Autodesk Inventor part; units mm, degrees
ref_plane "YZ Plane" through (0, 0, 0) normal (1, 0, 0) x (0, 1, 0)
ref_plane "XZ Plane" through (0, 0, 0) normal (0, 1, 0) x (-1, 0, 0)
ref_plane "XY Plane" through (0, 0, 0) normal (0, 0, 1) x (1, 0, 0)
sketch "Sketch1" plane through (0, 0, 0) normal (0, 0, 1) x (1, 0, 0)
  line L0 (1, -38.4) -> (1, -34.6)
  line L1 (1, -38.4) -> (20.6442, -38.4)
  line L2 (20.6442, -38.4) -> (20.6442, -34.6)
  line L3 (1, -34.6) -> (20.6442, -34.6)
  circle A0 centre (10.3221, -36.5) radius 1.0065
  line L4 (1, 0) -> (1, -3.8)
  line L5 (1, -3.8) -> (20.6442, -3.8)
  line L6 (20.6442, 0) -> (20.6442, -3.8)
  line L7 (1, 0) -> (20.6442, 0)
  circle A1 centre (10.3221, -1.9) radius 1.0065
  point P0 (0, 0)
extrude "Extrusion1" add sketch "Sketch1" along normal blind 4
sketch "Sketch2" plane through (0, 0, 4) normal (0, 0, 1) x (1, 0, 0)
  line L0 (20.6442, -34.6) -> (1, -34.6)
  line L1 (1, -34.6) -> (1, -38.4)
  line L2 (1, -38.4) -> (20.6442, -38.4)
  line L3 (20.6442, -38.4) -> (20.6442, -34.6)
  circle A0 centre (10.3221, -36.5) radius 1.0065
  line L4 (1, 0) -> (1, -3.8)
  line L5 (1, -3.8) -> (20.6442, -3.8)
  line L6 (20.6442, -3.8) -> (20.6442, 0)
  line L7 (20.6442, 0) -> (1, 0)
  circle A1 centre (10.3221, -1.9) radius 1.0065
  line L8 (1, -34.6) -> (1, -3.8)
  line L9 (20.6442, -3.8) -> (20.6442, -34.6)
  point P0 (0, 0)
extrude "Extrusion2" add sketch "Sketch2" against normal blind 1 contours L0 L8 L5 L9
sketch "Sketch3" plane through (1, 0, 0) normal (0, 1, 0) x (1, 0, 0)
  point P0 (-1, 0)
properties part number "PCBDownlHold"
CAD build for the part. Positions are in the model's coordinates, mm. A direction names the side the tool comes from. Give positions to 0.01 mm unless a question says otherwise; leave off trailing zeros. Loops run counter-clockwise (first coordinate to the right, second up) from the corner with the lowest first, then second, coordinate; pieces in that order, holes last. Notation, with made-up numbers: (85, 64) - (96, 64) arc R8 cw to (96, 68) - close; hole circle Ø11 at (23, 33). An arc over 180 degrees is marked (long way). Put each result on its own line as item: value.
Q1. Slice it at D-D (y = -6). Give the cut face in (x, z).
Filled in:
outline: (1, 3) - (20.64, 3) - (20.64, 4) - (1, 4) - close
Q2. Mould opens along Y. For faces 1 (the face through (10.7, -0.6, 0)), 2 (the face through (9.6, -37.2, 2)), 3 (the face through (11, -38.4, 2)), 4 (the face through (11, -3.8, 1)) say: pulls with the +Y half, pulls with the -Y half, needs draft (parallel to the pull), parting line crosses it, or undercut.
Filled in:
face 1: needs draft
face 2: undercut
face 3: pulls with the -Y half
face 4: undercut
Q3. Probe line 1 along Y through (x, z) = (3, 2.35); line 2 along Y through (x, z) = (9.75, 1.7); line 3 along Y through (x, z) = (10.75, 0.25). List the from-to ranges inside material, lowest first.
Filled in:
line 1: y = -38.4 to -34.6, -3.8 to 0
line 2: y = -38.4 to -37.33, -35.67 to -34.6, -3.8 to -2.73, -1.07 to 0
line 3: y = -38.4 to -37.41, -35.59 to -34.6, -3.8 to -2.81, -0.99 to 0
Q4. Slice it at A-A (y = -36.5). Give the cut face in (x, z).
Filled in:
outline: (1, 0) - (9.32, 0) - (9.32, 4) - (1, 4) - close; (11.33, 0) - (20.64, 0) - (20.64, 4) - (11.33, 4) - close
Q5. Tool access for faces 5 (the face through (11, -19, 3)), 6 (the face through (11, -38, 0)): list every direction of +Z, -Z, +X, -X, +Y, -Y with a clear straight run to the whole face (end or side of a thin tool).
Filled in:
face 5: -Z, +X, -X
face 6: -Z, +X, -X, +Y, -Y
Q6. Slice it at B-B (z = 2.35). Give the cut face in (x, y), plus the area to 3 significant figures.
Filled in:
outline: (1, -38.4) - (20.64, -38.4) - (20.64, -34.6) - (1, -34.6) - close; (1, -3.8) - (20.64, -3.8) - (20.64, 0) - (1, 0) - close; hole circle Ø2.01 at (10.32, -36.5); hole circle Ø2.01 at (10.32, -1.9)
area: 143 mm²
Q7. Slice it at C-C (x = 18.25). Give the cut face in (y, z), plus the area to 3 significant figures.
Filled in:
outline: (-38.4, 0) - (-34.6, 0) - (-34.6, 3) - (-3.8, 3) - (-3.8, 0) - (0, 0) - (0, 4) - (-38.4, 4) - close
area: 61.2 mm²
